```python
from build123d import *

# Parameters (mm, degrees)
BOARD_START         = 8.5
SKETCH1_R           = 1.25
BOARD_DEPTH         = 1.6
SERVO_START         = 10.1
SKETCH2_W           = 40.6
SKETCH2_H           = 7.6
SERVO_HEADERS_DEPTH = 11.5
V_START             = 10.1
SKETCH3_W           = 10
SKETCH3_H           = 7.5
V_TERMINAL_DEPTH    = 10
I2C_START           = 10.1
SKETCH4_W           = 2.5
SKETCH4_H           = 15.2
I2C_HEADERS_DEPTH   = 8.5


with BuildPart() as part:
    # Sketch1 → Board (new body)
    with BuildSketch(Plane(origin=(0, 0, 0), x_dir=(1, 0, 0), z_dir=(0, 1, 0)).offset(BOARD_START)):
        with BuildLine():
            Line((-30.1, 50.7), (30.1, 50.7))
            ThreePointArc((30.1, 50.7), (30.807106781, 50.407106781), (31.1, 49.7))
            Line((31.1, 49.7), (31.1, 26.3))
            ThreePointArc((31.1, 26.3), (30.807106781, 25.592893219), (30.1, 25.3))
            Line((30.1, 25.3), (-30.1, 25.3))
            ThreePointArc((-30.1, 25.3), (-30.807106781, 25.592893219), (-31.1, 26.3))
            Line((-31.1, 26.3), (-31.1, 49.7))
            ThreePointArc((-31.1, 49.7), (-30.807106781, 50.407106781), (-30.1, 50.7))
        make_face()
        with Locations(Location((-27.9, 47.5, 0), (0, 0, 270))):
            Circle(SKETCH1_R, mode=Mode.SUBTRACT)
        with Locations(Location((-27.9, 28.5, 0), (0, 0, 270))):
            Circle(SKETCH1_R, mode=Mode.SUBTRACT)
        with Locations(Location((27.9, 47.5, 0), (0, 0, 270))):
            Circle(SKETCH1_R, mode=Mode.SUBTRACT)
        with Locations(Location((27.9, 28.5, 0), (0, 0, 270))):
            Circle(SKETCH1_R, mode=Mode.SUBTRACT)
    extrude(amount=BOARD_DEPTH)

    # Sketch2 → Servo headers (add)
    with BuildSketch(Plane(origin=(0, 0, 0), x_dir=(1, 0, 0), z_dir=(0, 1, 0)).offset(SERVO_START)):
        with Locations((0, 30.5)):
            Rectangle(SKETCH2_W, SKETCH2_H)
    extrude(amount=SERVO_HEADERS_DEPTH)

    # Sketch3 → V+ terminal (add)
    with BuildSketch(Plane(origin=(0, 0, 0), x_dir=(1, 0, 0), z_dir=(0, 1, 0)).offset(V_START)):
        with Locations((0, 46.2)):
            Rectangle(SKETCH3_W, SKETCH3_H)
    extrude(amount=V_TERMINAL_DEPTH)

    # Sketch4 → I2C headers (add)
    with BuildSketch(Plane(origin=(0, 0, 0), x_dir=(1, 0, 0), z_dir=(0, 1, 0)).offset(I2C_START)):
        with Locations((-28.1, 38)):
            Rectangle(SKETCH4_W, SKETCH4_H)
        with Locations((28.1, 38)):
            Rectangle(SKETCH4_W, SKETCH4_H)
    extrude(amount=I2C_HEADERS_DEPTH)


solid = part.part
```
Build history of the part. All positions in model axes, mm. A direction names the side the tool comes from. Give positions to 0.01 mm unless a question says otherwise; leave off trailing zeros. Loops run counter-clockwise (first coordinate to the right, second up) from the corner with the lowest first, then second, coordinate; pieces in that order, holes last.
Item 1: Which spindle directions (+Z, -Z, +X, -X, +Y, -Y) get a long thin tool onto all of the face, cutting with end or side? Do faces 5 (the face through (-28, 18.6, -38)), 6 (the face through (0, 20.1, -46)), 7 (the face through (20.3, 16, -30)), 8 (the face through (0, 16, -34.3)). Say none if no direction does.
Answers follow:
face 5: +Z, -Z, -X, +Y
face 6: -Z, +X, -X, +Y
face 7: +Z, -Z, +Y
face 8: +Y
Item 2: Pull direction X, two halves, no side cores. Call faces 1 (the face through (0, 15, -49.95)), 2 (the face through (29.35, 14, -38)), 3 (the face through (-26.85, 14, -38)), 4 (the face through (-31.1, 9, -38)): released by +X, released by -X, zero draft, split by the parting line, or undercut.
Answers follow:
face 1: zero draft
face 2: released by +X
face 3: undercut
face 4: released by -X
Item 3: Drill centre lines: line 1 (X direction, y = 13, z = -44); line 2 (X direction, y = 9.4, z = -28.5); line 3 (X direction, y = 13.75, z = -34.75). Where is each one in solid material? Low to high.
Answers follow:
line 1: x = -29.35 to -26.85, -5 to 5, 26.85 to 29.35
line 2: x = -31.1 to -29.15, -26.65 to 26.65, 29.15 to 31.1
line 3: x = -29.35 to -26.85, 26.85 to 29.35
Item 4: Flat gauge pins, fed straight in: pin 1 (1.2 mm diameter, centred on x = -28, y = 13.5, fed in from +Z); pin 2 (1.5 mm diameter, centred on y = 11.5, z = -41.5, fed in from +X); pin 3 (4 mm diameter, centred on y = 18.5, z = -30.5, fed in from -X). Where does each tip first touch, or does it go through?
Answers follow:
pin 1: stops at z = -30.4
pin 2: stops at x = 29.35
pin 3: stops at x = -29.35
Item 5: Slice it at B-B, the plane x = -27.9. List the corners of the cut face in (y, z), and give its area (3 significant figures).
Answers follow:
outline: (8.5, -50.7) - (10.1, -50.7) - (10.1, -48.75) - (8.5, -48.75) - close; (8.5, -46.25) - (10.1, -46.25) - (10.1, -45.6) - (18.6, -45.6) - (18.6, -30.4) - (10.1, -30.4) - (10.1, -29.75) - (8.5, -29.75) - close; (8.5, -27.25) - (10.1, -27.25) - (10.1, -25.3) - (8.5, -25.3) - close
area: 162 mm2
Item 6: Slice it at C-C, the plane y = 17.5. List the corners of the cut face in (x, z), and give its area (3 significant figures).
Answers follow:
outline: (-29.35, -45.6) - (-26.85, -45.6) - (-26.85, -30.4) - (-29.35, -30.4) - close; (-20.3, -34.3) - (20.3, -34.3) - (20.3, -26.7) - (-20.3, -26.7) - close; (-5, -49.95) - (5, -49.95) - (5, -42.45) - (-5, -42.45) - close; (26.85, -45.6) - (29.35, -45.6) - (29.35, -30.4) - (26.85, -30.4) - close
area: 460 mm2
Item 7: Slice it at A-A, the plane z = -28.5. List the corners of the cut face in (x, y), and give its area (3 significant figures).
Answers follow:
outline: (-31.1, 8.5) - (-29.15, 8.5) - (-29.15, 10.1) - (-31.1, 10.1) - close; (-26.65, 8.5) - (26.65, 8.5) - (26.65, 10.1) - (20.3, 10.1) - (20.3, 21.6) - (-20.3, 21.6) - (-20.3, 10.1) - (-26.65, 10.1) - close; (29.15, 8.5) - (31.1, 8.5) - (31.1, 10.1) - (29.15, 10.1) - close
area: 558 mm2
Item 8: Slice it at D-D, the plane z = -38.5. List the corners of the cut face in (x, y), and give its area (3 significant figures).
Answers follow:
outline: (-31.1, 8.5) - (31.1, 8.5) - (31.1, 10.1) - (29.35, 10.1) - (29.35, 18.6) - (26.85, 18.6) - (26.85, 10.1) - (-26.85, 10.1) - (-26.85, 18.6) - (-29.35, 18.6) - (-29.35, 10.1) - (-31.1, 10.1) - close
area: 142 mm2
